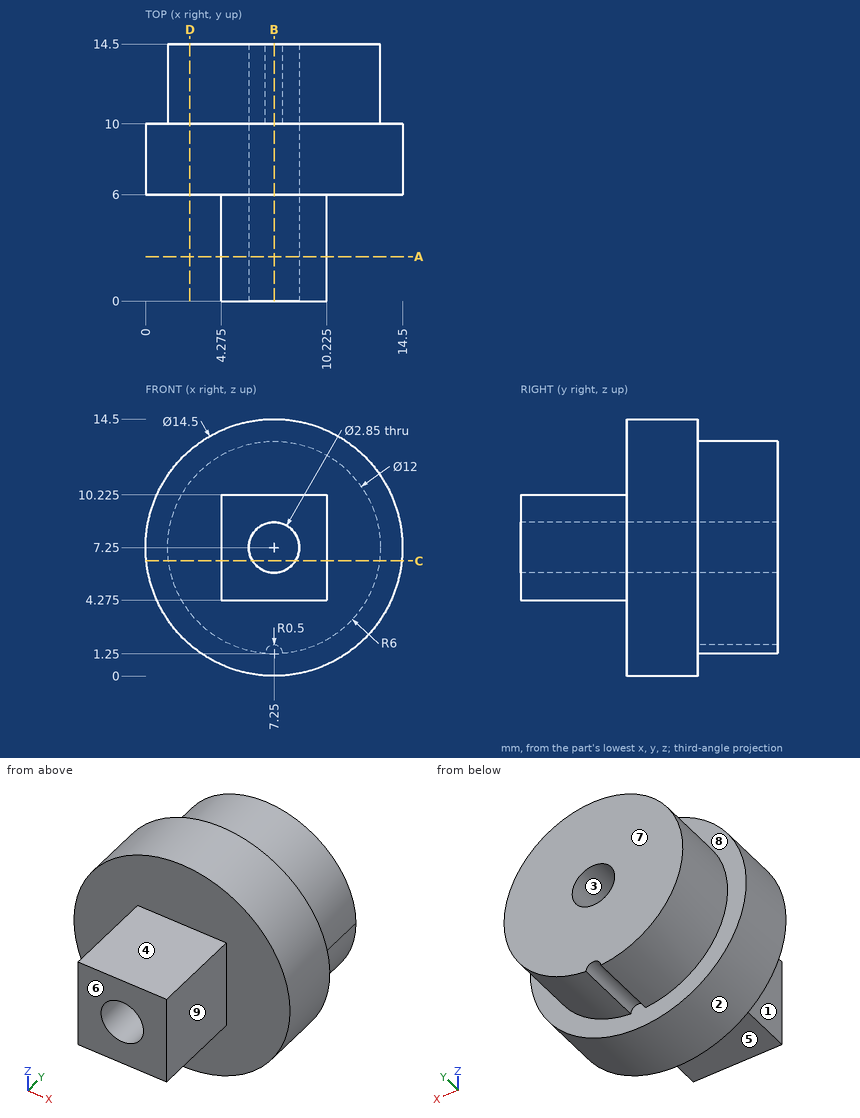
Can you work these out from the drawing? Everything is in mm from the part's minimum corner. A direction names the side the tool comes from. Give positions to 0.01 mm unless a question says otherwise; leave off trailing zeros. Loops run counter-clockwise (first coordinate to the right, second up) from the corner with the lowest first, then second, coordinate; pieces in that order, holes last. Notation, with made-up numbers: (61, 42) - (89, 42) arc R25 ccw to (89, 56) - close; hole circle Ø3 at (22.5, 82). An arc over 180 degrees is marked (long way). Use one line per item in the form item = value.
1. I need wall thicknesses on probe 1 along Z at (x, y) = (7.25, 3.75) (3 decimals); probe 2 along X at (y, z) = (8.25, 7.25) (3 decimals). Which ranges of each line are inside material? Lowest first, please.
Response values:
probe_1 = 4.275 to 5.825, 8.675 to 10.225
probe_2 = 0 to 5.825, 8.675 to 14.5
2. On a 3-axis mill with a long thin cutter (end or side, diameter ignored), from which of +Z, -Z, +X, -X, +Y, -Y can I reach the whole of each face in a straight line? I mean the marked faces 5, 6, 7, 8 and 9. Say none if no direction works.
Response values:
face_5 = -Z, +X, -X, -Y
face_6 = +Z, -Z, +X, -X, -Y
face_7 = +Z, -Z, +X, -X, +Y
face_8 = +Y
face_9 = +Z, -Z, +X, -Y
3. Thinking about a two-plate mould opening in X: for the marked faces 1, 2, 3 and 4, which applies, released by +X, released by -X, zero draft, split by the parting line, or undercut?
Response values:
face_1 = released by -X
face_2 = split by the parting line
face_3 = undercut
face_4 = zero draft
4. I want a section at B-B (x = 7.25). Please give me the cut outline in (y, z) (3 decimals), and give its area (3 significant figures).
Response values:
outline = (0, 4.275) - (6, 4.275) - (6, 0) - (10, 0) - (10, 1.75) - (14.5, 1.75) - (14.5, 5.825) - (0, 5.825) - close; (0, 8.675) - (14.5, 8.675) - (14.5, 13.25) - (10, 13.25) - (10, 14.5) - (6, 14.5) - (6, 10.225) - (0, 10.225) - close
area = 104 mm²
5. I want a section at D-D (x = 2.5). Please give me the cut outline in (y, z), and give its area (3 significant figures).
Response values:
outline = (6, 1.77) - (10, 1.77) - (10, 3.58) - (14.5, 3.58) - (14.5, 10.92) - (10, 10.92) - (10, 12.73) - (6, 12.73) - close
area = 76.8 mm²
6. I want a section at A-A (y = 2.5). Please give me the cut outline in (x, z) (3 decimals).
Response values:
outline = (4.275, 4.275) - (10.225, 4.275) - (10.225, 10.225) - (4.275, 10.225) - close; hole circle Ø2.85 at (7.25, 7.25)
7. I'm going to push flat-ended pins straight in: pin 1 Ø5 at (y, z) = (12, 13) entering from +X; pin 2 Ø3 at (y, z) = (3, 8) entering from -X (3 decimals); pin 3 Ø2 at (x, y) = (8.5, 2.5) entering from -Z (3 decimals); pin 4 Ø4.5 at (x, z) = (9, 6.5) entering from -Y. Where does each tip first touch, or does it pass through?
Response values:
pin_1 = 13.12
pin_2 = 4.275
pin_3 = 4.275
pin_4 = 0
8. I want a section at C-C (z = 6.5). Please give me the cut outline in (x, y) (3 decimals), and give its area (3 significant figures).
Response values:
outline = (0.039, 6) - (4.275, 6) - (4.275, 0) - (6.038, 0) - (6.038, 14.5) - (1.297, 14.5) - (1.297, 10) - (0.039, 10) - close; (8.462, 0) - (10.225, 0) - (10.225, 6) - (14.461, 6) - (14.461, 10) - (13.203, 10) - (13.203, 14.5) - (8.462, 14.5) - close
area = 112 mm²
